Check sheet for the modelled part. Datum: model origin and axes. Units: mm. A direction names the side the tool comes from. Coordinates: 2 decimals unless noted, no trailing zeros. Write each loop counter-clockwise with the first axis right and the second up, starting at its lowest first coordinate (ties: lowest second). Pieces come first, ordered by that corner, then holes. Notation, with made-up numbers: M -12.75,31.5 L 27.25,31.5 A19 ccw 27.25,40.5 Z; hole C 47,46 d1. An arc over 180 degrees is marked long. Answer as CSV lines item,"result". Start each with the question number.
Q1. Depth check by flat-ended pin: pin 1 Ø0.8 at (y, z) = (15, 0.5) entering from +X; pin 2 Ø1.5 at (y, z) = (9, -0.5) entering from -X; pin 3 Ø1 at (x, y) = (1, 9.5) entering from +Z. Enter the tip coordinate at first touch or a pass-through.
Q2. Mould release check, pull along X, two halves, no side actions. Record for faces 3 (the cylindrical face through (1.5, 6.16, -0.07)), 4 (the flat face through (0, 0, 0)), 5 (the flat face through (0, 14.5, 0)): pulls with the +X half, pulls with the -X half, needs draft (parallel to the pull), parting line crosses it, or undercut.
Q3. Access from +Z, -Z, +X, -X, +Y, -Y to the whole of each face (thin tool, end or side, straight path). Record for faces 1 (the cylindrical face through (-0.33, 13.99, 2.52)), 2 (the flat face through (-0.66, 15.01, 1.12)).
Q4. Thickness scan on line 1 along Y through (x, z) = (1.5, 0.4); line 2 along Y through (x, z) = (0.7, 0.65); line 3 along Z through (x, y) = (0.1, 12). Record the ranges inside material, lowest first. Write a range as from..to.
Q5. Sectioned sample at A-A, the plane z = 0. Record the cut outline in (x, y), then the cut area to 3 significant figures.
Q6. Sectioned sample at B-B, the plane y = 2.25. Record the cut outline in (x, z), then the cut area to 3 significant figures.
Autodesk Inventor part; units mm, degrees
ref_plane "YZ Plane" through (0, 0, 0) normal (1, 0, 0) x (0, 1, 0)
ref_plane "XZ Plane" through (0, 0, 0) normal (0, 1, 0) x (-1, 0, 0)
ref_plane "XY Plane" through (0, 0, 0) normal (0, 0, 1) x (1, 0, 0)
sketch "Sketch1" plane through (0, 0, 0) normal (0, 1, 0) x (-1, 0, 0)
  circle A0 centre (0, 0) radius 1.5
  dimension "d0" = 3
extrude "Extrusion1" add sketch "Sketch1" along normal blind 12.5
sketch "Sketch2" plane through (0, 12.5, 0) normal (0, 1, 0) x (1, 0, 0)
  circle A0 centre (0, 0) radius 1.5
  circle A1 centre (0, 0) radius 2.54
  dimension "d3" = 5.08
extrude "Extrusion2" add sketch "Sketch2" along normal blind 3 contours A0 | A1
fillet "Fillet1" radius 0.508 2 edges at (-2.54, 15.5, 0) (-2.54, 12.5, 0)
sketch "Sketch3" plane through (0, 15.5, 0) normal (0, 1, 0) x (1, 0, 0)
  line L0 (0, 0) -> (1.5, 0) construction
  line L1 (-1.299, -0.75) -> (-1.299, 0.75)
  line L2 (-1.299, 0.75) -> (0.0002, 1.5)
  line L3 (1.299, 0.75) -> (0.0002, 1.5)
  line L4 (1.299, 0.75) -> (1.299, -0.75)
  line L5 (0, -1.5) -> (1.299, -0.75)
  line L6 (-1.299, -0.75) -> (0, -1.5)
thread "Thread1"
extrude "Extrusion4" cut sketch "Sketch3" against normal blind 1
properties part number "screw"
Output:
1,pin 1,"stops at x = 2.54"
1,pin 2,"stops at x = -1.5"
1,pin 3,"stops at z = 1.41"
2,face 3,"parting line crosses it"
2,face 4,"needs draft"
2,face 5,"undercut"
3,face 1,"+Y, -Y"
3,face 2,"+Y"
4,line 1,"y = 12.5..15.5"
4,line 2,"y = 0..14.5"
4,line 3,"z = -1.5..1.5"
5,outline,"M -2.54,13.01 A0.51 ccw -2.03,12.5 L -1.5,12.5 L -1.5,0 L 1.5,0 L 1.5,12.5 L 2.03,12.5 A0.51 ccw 2.54,13.01 L 2.54,14.99 A0.51 ccw 2.03,15.5 L 1.3,15.5 L 1.3,14.5 L -1.3,14.5 L -1.3,15.5 L -2.03,15.5 A0.51 ccw -2.54,14.99 Z"
5,area,"49.9 mm^2"
6,outline,"C 0,0 d3"
6,area,"7.07 mm^2"
